The figure shows three views and two pictorial views of one solid part (mm, origin at its lowest corner). Answer the questions. A direction names the side the tool comes from. Coordinates: 2 decimals unless noted, no trailing zeros. Loops run counter-clockwise (first coordinate to the right, second up) from the corner with the lowest first, then second, coordinate; pieces in that order, holes last. Notation, with made-up numbers: M -25.5,26 L 26.5,26 A25 cw 26.5,62 Z; hole C 1,87.25 d11. An arc over 180 degrees is marked long. One line per item, written item: value. Start each with the question number.
1. The part is cut by section C-C (x = 147). Write down the section's boundary in (y, z).
2. For the marked faces 1 and 2, determine the directions among +Z, -Z, +X, -X, +Y, -Y from which every point of the face is accessible in a straight line to the end or side of a thin tool.
3. The part is cut by section B-B (z = 141.5). Write down the section's boundary in (x, y), then the cut area to 3 significant figures.
4. The part is cut by section A-A (y = 9.25). Write down the section's boundary in (x, z), then the cut area to 3 significant figures.
5. The part is cut by section D-D (z = 28). Write down the section's boundary in (x, y), then the cut area to 3 significant figures.
6. Consider probe 1 along Z at (x, y) = (50, 2.1); probe 2 along Z at (x, y) = (80, 14.25); probe 3 along Y at (x, z) = (14, 137.7). Determine where each line is inside the solid, lowest interval first.
7. Determine the mould class of the marked faces 3, 4 and 5 for opening direction Z: +Z half, -Z half, draft (parallel to the pull), parting line (faces both ways), or undercut.
8. Flat-ended cylindrical pins translate along their axes: pin 1 (16.5 mm diameter, centred on x = 125, z = 147.5, fed in from +Y); pin 2 (2 mm diameter, centred on x = 134.5, y = 13, fed in from -Z); pin 3 (5.5 mm diameter, centred on x = 164, y = 14.922, fed in from +Z). Find the tip coordinate at first contact, or state that the pin passes through.
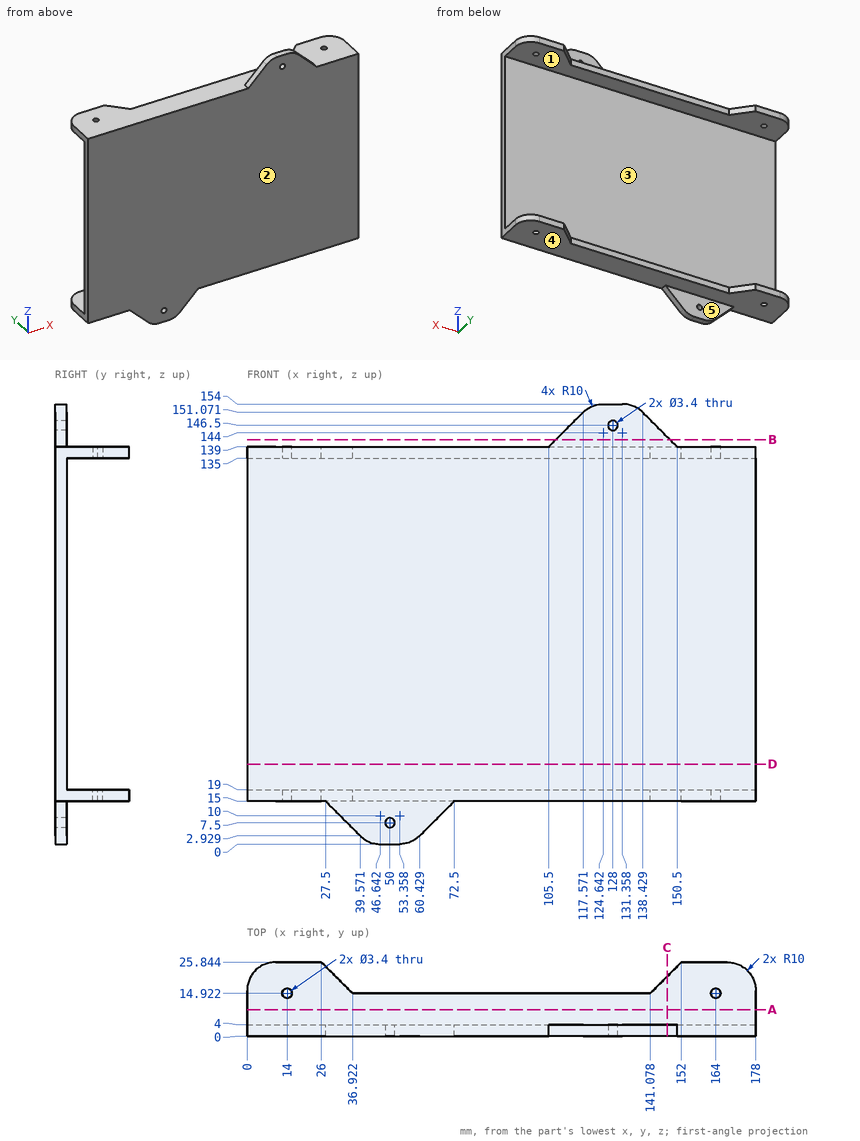
Answer block:
1. outline: M 0,15 L 20.84,15 L 20.84,19 L 4,19 L 4,135 L 20.84,135 L 20.84,139 L 4,139 L 4,142.5 L 0,142.5 Z
2. face 1: +X, -X, +Y
2. face 2: +Z, -Z, +X, -X, -Y
3. outline: M 108,0 L 148,0 L 148,4 L 108,4 Z
3. area: 160 mm2
4. outline: M 0,15 L 178,15 L 178,19 L 0,19 Z; M 0,135 L 178,135 L 178,139 L 0,139 Z
4. area: 1,420 mm2
5. outline: M 0,0 L 178,0 L 178,4 L 0,4 Z
5. area: 712 mm2
6. probe 1: z = 0 to 5.8, 9.2 to 139
6. probe 2: z = 15 to 19, 135 to 139
6. probe 3: y = 0 to 13.22, 16.62 to 25.84
7. face 3: undercut
7. face 4: -Z half
7. face 5: draft
8. pin 1: stops at y = 4
8. pin 2: stops at z = 15
8. pin 3: stops at z = 139
